Autodesk Inventor part; units mm, degrees
ref_plane "YZ Plane" through (0, 0, 0) normal (1, 0, 0) x (0, 1, 0)
ref_plane "XZ Plane" through (0, 0, 0) normal (0, 1, 0) x (-1, 0, 0)
ref_plane "XY Plane" through (0, 0, 0) normal (0, 0, 1) x (1, 0, 0)
sketch "Sketch1" plane through (0, 0, 0) normal (0, 0, 1) x (1, 0, 0)
  ellipse E0 centre (0, 0) end of major axis (-17.5, 0) minor radius 2.5
  line L0 (0, 0) -> (0, -2.5)
  dimension "d0" = 17.5
  dimension "d1" = 2.5
extrude "Extrusion1" add sketch "Sketch1" along normal mid plane 1
sketch "Sketch2" plane through (0, 0, 0.5) normal (0, 0, 1) x (1, 0, 0)
  ellipse E0 centre (0, 0) end of major axis (17.5, 0) minor radius 2.5
  circle A0 centre (0, 0) radius 3
  dimension "d4" = 6
extrude "Extrusion2" add sketch "Sketch2" along normal blind 2 and the other way blind 1 contours A0 E0 | E0 A0 | A0 E0 picked at (1.5591, 0) picked at (0.3978, 2.6587) picked at (0.3978, -2.6587)
sketch "Sketch3" plane through (0, 0, 2.5) normal (0, 0, 1) x (1, 0, 0)
  circle A0 centre (0, 0) radius 3
  circle A1 centre (0, 0) radius 2.5
  dimension "d7" = 5
extrude "Extrusion3" cut sketch "Sketch3" against normal blind 2 contours A1
sketch "Sketch4" plane through (0, 0, -0.5) normal (0, 0, -1) x (-1, 0, 0)
  ellipse E0 centre (0, 0) end of major axis (-17.5, 0) minor radius 2.5
  circle A0 centre (0, 0) radius 2
  dimension "d10" = 4
extrude "Extrusion4" cut sketch "Sketch4" against normal blind 0.5 contours A0
sketch "Sketch5" plane through (0, 0, 0) normal (0, 0, -1) x (-1, 0, 0)
  circle A0 centre (0, 0) radius 2
  circle A1 centre (0, 0) radius 1
  dimension "d13" = 2
extrude "Extrusion5" cut sketch "Sketch5" against normal through all contours A1
sketch "Sketch6" plane through (0, 0, -0.5) normal (0, 0, -1) x (-1, 0, 0)
  ellipse E0 centre (0, 0) end of major axis (-17.5, 0) minor radius 2.5
  circle A0 centre (-16, 0) radius 0.5
  line L0 (0, 0) -> (0, -1.2687)
  line L1 (0, 0) -> (-1.4808, 0)
  dimension "d16" = 1
  dimension "d17" = 16
extrude "Extrusion6" cut sketch "Sketch6" against normal through all contours A0
pattern_linear "Rectangular Pattern1" count 6 spacing 2.5 along (-1, 0, 0) of "Extrusion6"
mirror "Mirror2" about plane through (0, 0, 0) normal (1, 0, 0) of "Extrusion6", "Rectangular Pattern1"
sketch "Sketch7" plane through (0, 0, -0.5) normal (0, 0, -1) x (-1, 0, 0)
  circle A0 centre (0, 0) radius 2
  arc A1 (1.6755, 2.4885) -> (-1.6755, 2.4885) centre (0, 0) ccw
  line L0 (2, -7) -> (-2, -7)
  line L1 (-2, -7) -> (-2, 7)
  line L2 (-2, 7) -> (2, 7)
  line L3 (2, 7) -> (2, -7)
  line L4 (0, 0) -> (0, 1.4793)
  line L5 (0, 0) -> (-1.001, 0)
  circle A2 centre (0, 7) radius 2
  circle A3 centre (0, -7) radius 2
  circle A4 centre (0, 0) radius 2
  point P0 (2, 0)
  dimension "d25" = 4
  dimension "d26" = 14
extrude "Extrusion7" add sketch "Sketch7" against normal blind 1 contours L3 A3 L1 A0 | A0 L1 A2 L3 | A2 L2 | L2 A2 | A3 L0 | L0 A3
sketch "Sketch8" plane through (0, 0, -0.5) normal (0, 0, -1) x (-1, 0, 0)
  arc A0 (2, 7) -> (-2, 7) centre (0, 7) ccw
  circle A1 centre (0, 7) radius 0.5
  dimension "d29" = 1
extrude "Extrusion8" cut sketch "Sketch8" against normal blind 1
pattern_linear "Rectangular Pattern2" count 2 spacing 3 along (0, -1, 0) of "Extrusion8"
mirror "Mirror3" about plane through (0, 0, 0) normal (0, 1, 0) of "Extrusion8", "Rectangular Pattern2"
properties material "PVC-Piping"
Verification items for the finished model (mm, model axes). A direction names the side the tool comes from. Coordinates: 2 decimals unless noted, no trailing zeros. Order: outer loops, then holes, each group sorted by start corner. A loop starts at its lowest first (then second) coordinate and runs counter-clockwise, first axis right, second up.
1. Set-up check for faces 1 (the face through (2, -5, 0)), 2 (the face through (1, -1, 0.5)), 3 (the face through (-1, -1, 0)), 4 (the face through (-2, -5, 0)): record each of +Z, -Z, +X, -X, +Y, -Y from which the full face is reachable in a straight line by a thin tool's end or side.
Results found:
face 1: +Z, -Z, +X, -Y
face 2: +Z
face 3: -Z
face 4: +Z, -Z, -X, -Y
2. Sectioned sample at A-A, the plane z = 1.15. Record the cut outline in (x, y), and give its area (3 significant figures).
Results found:
outline: circle Ø6 at (0, 0); hole circle Ø5 at (0, 0)
area: 8.64 mm2
3. Go/stop test with flat-tipped pins: pin 1 Ø3 at (x, y) = (0, 0) entering from +Z; pin 2 Ø0.8 at (y, z) = (-4.5, 0) entering from +X; pin 3 Ø0.8 at (y, z) = (-4.5, 0) entering from -X. Record where each tip stops, or that it passes through.
Results found:
pin 1: stops at z = 0.5
pin 2: stops at x = 2
pin 3: stops at x = -2
4. Sectioned sample at B-B, the plane x = 1.5. Record the cut outline in (y, z).
Results found:
outline: (-8.32, -0.5) - (-1.32, -0.5) - (-1.32, 0) - (1.32, 0) - (1.32, -0.5) - (8.32, -0.5) - (8.32, 0.5) - (2.6, 0.5) - (2.6, 2.5) - (2, 2.5) - (2, 0.5) - (-2, 0.5) - (-2, 2.5) - (-2.6, 2.5) - (-2.6, 0.5) - (-8.32, 0.5) - close
5. Release check for a two-part mould opening along X. For faces 5 (the face through (-2, 5, 0)), 6 (the face through (-3, 0, 2)), 7 (the face through (2, 5, 0)), 8 (the face through (8, 0, 0)) record: +X half, -X half, draft (parallel to the pull), parting line (faces both ways), or undercut.
Results found:
face 5: -X half
face 6: parting line
face 7: +X half
face 8: undercut
6. Scan lines: line 1 (Y direction, x = 0, z = 0.05); line 2 (Y direction, x = 0, z = 1.95); line 3 (Z direction, x = 10.5, y = 1.5). Record each from-to range of solid material in increasing order.
Results found:
line 1: y = -9 to -7.5, -6.5 to -4.5, -3.5 to -1, 1 to 3.5, 4.5 to 6.5, 7.5 to 9
line 2: y = -3 to -2.5, 2.5 to 3
line 3: z = -0.5 to 0.5
